Verification items for this drawing (mm, ordinates from the low corner). A direction names the side the tool comes from. Coordinates: 2 decimals unless noted, no trailing zeros. Order: outer loops, then holes, each group sorted by start corner. A loop starts at its lowest first (then second) coordinate and runs counter-clockwise, first axis right, second up. Notation, with made-up numbers: M -13.5,56 L 28.5,56 A28 cw 28.5,76 Z; hole C 72,-0.75 d5. An arc over 180 degrees is marked long. Answer as a JSON object with one key per item and string values. Group by question number.
(1) Cross-section at C-C (x = 14.25). Enter the section's corners in (y, z), plus the area to 3 significant figures.
(2) Cross-section at D-D (y = 9). Enter the section's corners in (x, z), plus the area to 3 significant figures.
(3) Material ranges on line 1 (Z direction, x = 5.75, y = 10.7); line 2 (Z direction, x = 12, y = 6); line 3 (Z direction, x = 10.5, y = 10.75), recorded low to high.
(4) Mould release check, pull along Y, two halves, no side actions. Record for the marked faces 3, 4 and 5: released by +Y, released by -Y, zero draft, split by the parting line, or undercut.
(5) Access from +Z, -Z, +X, -X, +Y, -Y to the whole of each face (thin tool, end or side, straight path). Record for the marked faces 1 and 2.
(6) Cross-section at A-A (x = 6.25). Enter the section's corners in (y, z), plus the area to 3 significant figures.
(7) Cross-section at B-B (z = 7.75). Enter the section's corners in (x, y), plus the area to 3 significant figures.
(8) Gauge pin test, flat ends, axial feed: pin 1 Ø2.5 at (x, y) = (8.5, 1) entering from +Z; pin 2 Ø6 at (x, z) = (11.5, 4.5) entering from -Y; pin 3 Ø1.3 at (y, z) = (11, 7) entering from -X; pin 4 Ø3 at (x, z) = (11.5, 8) entering from -Y. Record the tip position at first contact, or that the pin passes through.
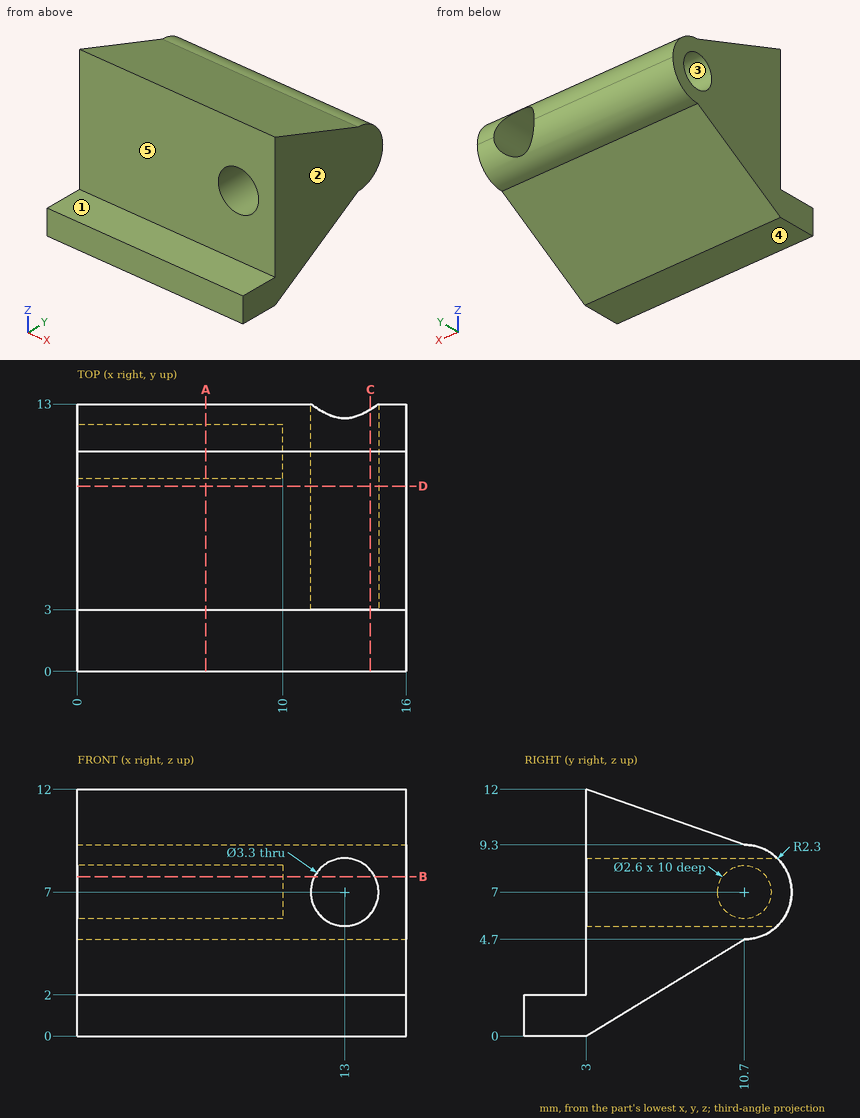
Taken from the geometry:
{
 "1": {"outline": "M 0,0 L 3,0 L 10.7,4.7 A2.3 ccw 12.73,5.92 L 3,5.92 L 3,2 L 0,2 Z; M 3,8.08 L 12.73,8.08 A2.3 ccw 10.7,9.3 L 3,12 Z", "area": "56.9 mm²"},
 "2": {"outline": "M 0,3.66 L 16,3.66 L 16,9.9 L 0,9.9 Z; hole C 13,7 d3.3", "area": "91.2 mm²"},
 "3": {"line 1": "z = 4.7 to 5.7, 8.3 to 9.3", "line 2": "z = 1.83 to 5.69, 8.31 to 10.95", "line 3": "z = 4.7 to 9.3"},
 "4": {"face 3": "undercut", "face 4": "zero draft", "face 5": "released by -Y"},
 "5": {"face 1": "+Z, +X, -X, -Y", "face 2": "+Z, -Z, +X, +Y, -Y"},
 "6": {"outline": "M 0,0 L 3,0 L 10.7,4.7 A2.3 ccw 13,7 A2.3 ccw 10.7,9.3 L 3,12 L 3,2 L 0,2 Z; hole C 10.7,7 d2.6", "area": "72.9 mm²"},
 "7": {"outline": "M 0,3 L 11.53,3 L 11.53,12.87 L 0,12.87 L 0,11.76 L 10,11.76 L 10,9.64 L 0,9.64 Z; M 14.47,3 L 16,3 L 16,12.87 L 14.47,12.87 Z", "area": "108 mm²"},
 "8": {"pin 1": "stops at z = 2", "pin 2": "stops at y = 0", "pin 3": "stops at x = 10", "pin 4": "stops at y = 3"}
}
